Answer from the drawing. Dimensions are ordinates in mm from the lowest x, y and z of the part. A direction names the side the tool comes from. Coordinates: 2 decimals unless noted, no trailing zeros. Write each loop counter-clockwise with the first axis right and the second up, starting at its lowest first coordinate (ties: lowest second). Pieces come first, ordered by that corner, then holes. Notation, with made-up numbers: (86.5, 10.25) -> (97.5, 10.25) arc R31 ccw to (97.5, 49.25) -> close; hole circle Ø3 at (33, -24). An arc over 180 degrees is marked (long way). Use CSV: the item, a comma, the result in double quotes.
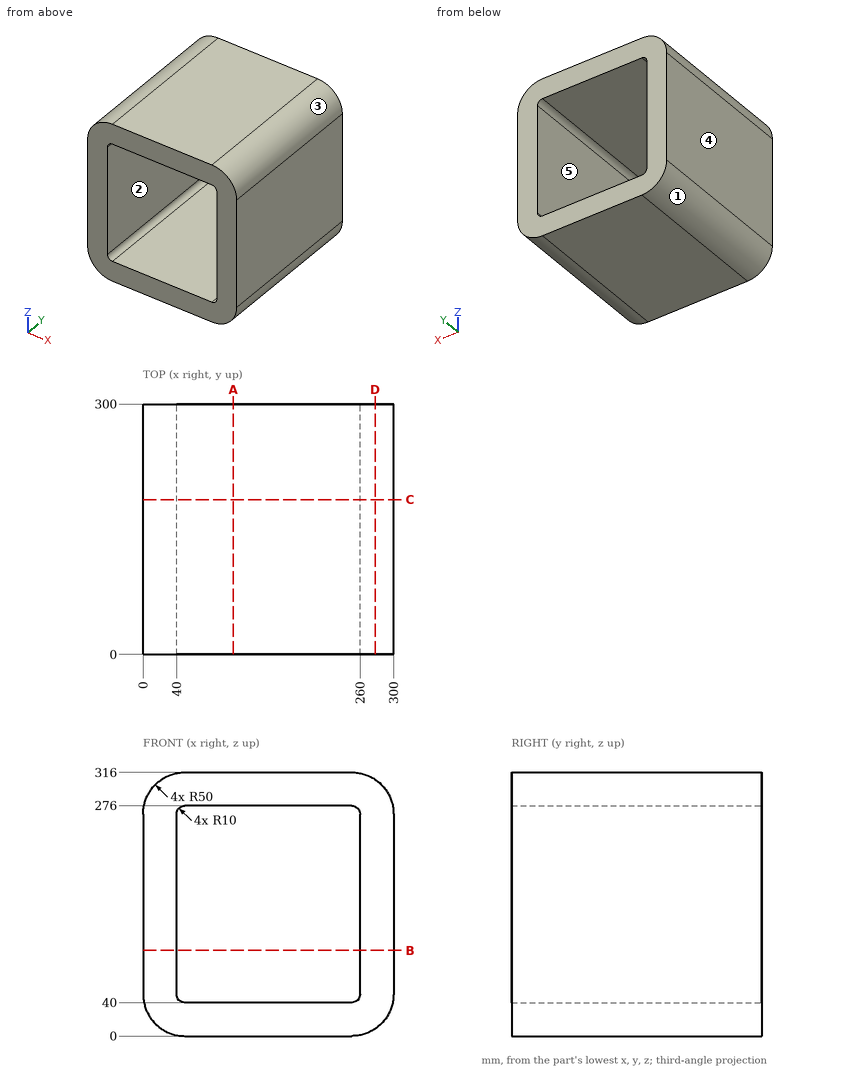
1. A cutting plane is placed at D-D (x = 278). Give the vertices of the cut face in (y, z), and give its area (3 significant figures).
Solutions:
outline,"(0, 8.58) -> (300, 8.58) -> (300, 307.42) -> (0, 307.42) -> close"
area,"89,700 mm^2"
2. A cutting plane is placed at C-C (y = 185.5). Give the vertices of the cut face in (x, z), and give its area (3 significant figures).
Solutions:
outline,"(0, 50) arc R50 ccw to (50, 0) -> (250, 0) arc R50 ccw to (300, 50) -> (300, 266) arc R50 ccw to (250, 316) -> (50, 316) arc R50 ccw to (0, 266) -> close; hole (40, 50) arc R10 ccw to (50, 40) -> (250, 40) arc R10 ccw to (260, 50) -> (260, 266) arc R10 ccw to (250, 276) -> (50, 276) arc R10 ccw to (40, 266) -> close"
area,"40,800 mm^2"
3. For a pull along X with two mould halves and no side action, classify the marked faces 3, 4 and 5 as pulls with the +X half, pulls with the -X half, needs draft (parallel to the pull), parting line crosses it, or undercut.
Solutions:
face 3,"pulls with the +X half"
face 4,"pulls with the -X half"
face 5,"undercut"
4. A cutting plane is placed at A-A (x = 108). Give the vertices of the cut face in (y, z), and give its area (3 significant figures).
Solutions:
outline,"(0, 0) -> (300, 0) -> (300, 40) -> (0, 40) -> close; (0, 276) -> (300, 276) -> (300, 316) -> (0, 316) -> close"
area,"24,000 mm^2"
5. A cutting plane is placed at B-B (z = 102.5). Give the vertices of the cut face in (x, y), and give its area (3 significant figures).
Solutions:
outline,"(0, 0) -> (40, 0) -> (40, 300) -> (0, 300) -> close; (260, 0) -> (300, 0) -> (300, 300) -> (260, 300) -> close"
area,"24,000 mm^2"
6. A tool of negligible diameter and unlimited length cuts with its end or side. For the marked faces 1 and 2, from which of +Z, -Z, +X, -X, +Y, -Y can it reach the whole face along a straight path? Write none if from no direction.
Solutions:
face 1,"-Z, -X, +Y, -Y"
face 2,"+Y, -Y"
7. Find the intervals of material crossed by line 1 along Z through (x, y) = (72, 224.5); line 2 along X through (y, z) = (204, 75); line 3 along X through (y, z) = (227, 283), in increasing order.
Solutions:
line 1,"z = 0 to 40, 276 to 316"
line 2,"x = 0 to 40, 260 to 300"
line 3,"x = 2.98 to 297.02"
